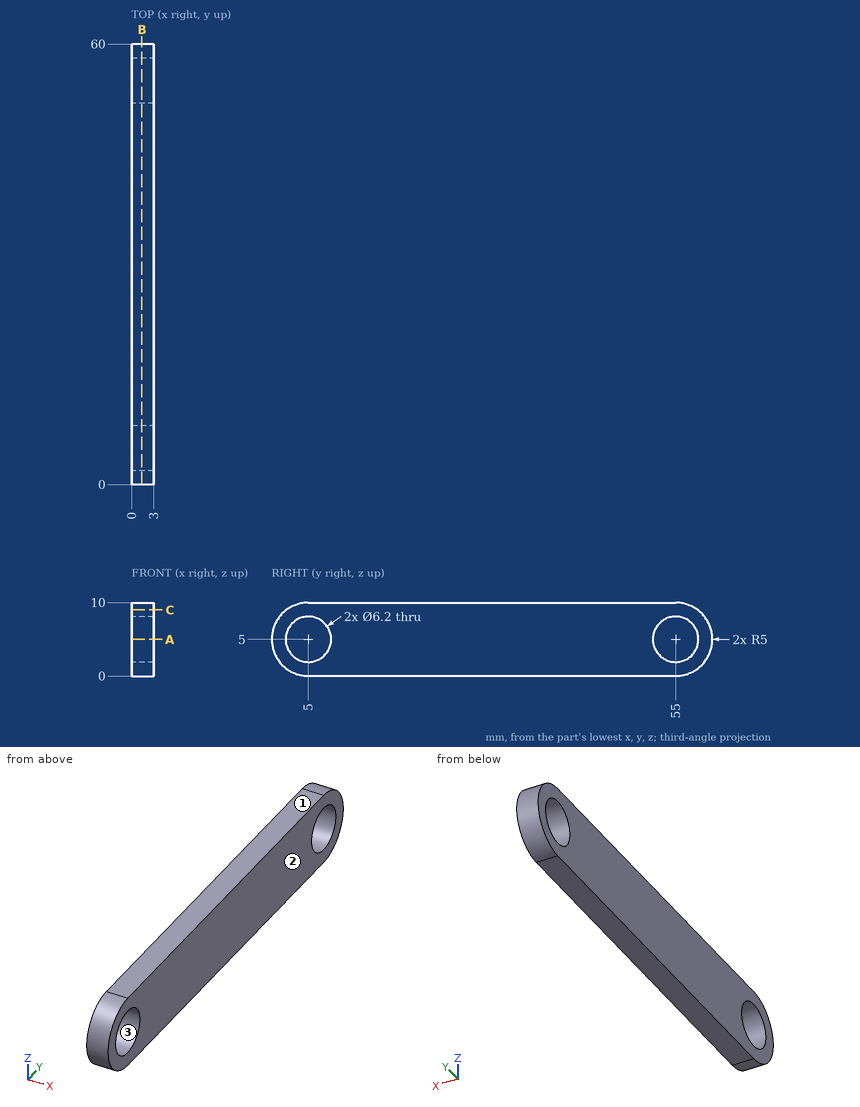
The drawing under review shows one solid part. Ordinate dimensions are in mm from its lowest x, y, z. Coordinates: 2 decimals unless noted, no trailing zeros. Order: outer loops, then holes, each group sorted by start corner. A loop starts at its lowest first (then second) coordinate and runs counter-clockwise, first axis right, second up. Notation, with made-up numbers: (-29, 31.5) -> (22, 31.5) arc R10 cw to (22, 49.5) -> close; hole circle Ø9 at (37.25, -29). An arc over 180 degrees is marked (long way). One line per item, written item: value.
1) We need section A-A, the plane z = 5. Give the boundary of the cut face in (x, y), then the cut area to 3 significant figures.
Output values:
outline: (0, 0) -> (3, 0) -> (3, 1.9) -> (0, 1.9) -> close; (0, 8.1) -> (3, 8.1) -> (3, 51.9) -> (0, 51.9) -> close; (0, 58.1) -> (3, 58.1) -> (3, 60) -> (0, 60) -> close
area: 143 mm2
2) We need section C-C, the plane z = 9. Give the boundary of the cut face in (x, y).
Output values:
outline: (0, 2) -> (3, 2) -> (3, 58) -> (0, 58) -> close
3) We need section B-B, the plane x = 1.4. Give the boundary of the cut face in (y, z).
Output values:
outline: (5, 0) -> (55, 0) arc R5 ccw to (55, 10) -> (5, 10) arc R5 ccw to start; hole circle Ø6.2 at (5, 5); hole circle Ø6.2 at (55, 5)
4) To check wall thickness, follow probe 1 along Y at (x, z) = (2.1, 2.5); probe 2 along Z at (x, y) = (0.95, 5); probe 3 along Y at (x, z) = (0.6, 6.75). State the ranges of each line that lie inside material, in increasing order. Write a range as [from, to].
Output values:
probe 1: y = [0.67, 3.17], [6.83, 53.17], [56.83, 59.33]
probe 2: z = [0, 1.9], [8.1, 10]
probe 3: y = [0.32, 2.44], [7.56, 52.44], [57.56, 59.68]
5) Draft analysis for pull direction Z (two halves, no side actions). For the marked faces 1, 2 and 3, state which applies: +Z half, -Z half, draft (parallel to the pull), parting line (faces both ways), or undercut.
Output values:
face 1: +Z half
face 2: draft
face 3: undercut
6) Clearance check with flat-ended pins moving along their axes: P1, Ø1.5, axis at x = 2, y = 30, coming from the -Z side; P2, Ø1, axis at x = 2, z = 3, coming from the -Y side; P3, Ø5, axis at y = 55, z = 5, coming from the +X side. State where each tip first meets the part, or that it passes through.
Output values:
P1: stops at z = 0
P2: stops at y = 0.23
P3: passes through
